Model file for the job. Use its own axes, mm. Face numbers are marked on the shaded views. A direction names the side the tool comes from. Give positions to 0.01 mm unless a question says otherwise; leave off trailing zeros. Loops run counter-clockwise (first coordinate to the right, second up) from the corner with the lowest first, then second, coordinate; pieces in that order, holes last. Notation, with made-up numbers: M 19.5,-31 L 46.5,-31 A9 ccw 46.5,-21 Z; hole C 3,-18 d6. An arc over 180 degrees is marked long. Answer in a Markdown table with one row per item.
Autodesk Inventor part; units mm, degrees
ref_plane "YZ Plane" through (0, 0, 0) normal (1, 0, 0) x (0, 1, 0)
ref_plane "XZ Plane" through (0, 0, 0) normal (0, 1, 0) x (-1, 0, 0)
ref_plane "XY Plane" through (0, 0, 0) normal (0, 0, 1) x (1, 0, 0)
sketch "Sketch1" plane through (0, 0, 0) normal (0, 1, 0) x (-1, 0, 0)
  line L0 (-10, 10) -> (10, 10)
  line L1 (10, 10) -> (10, -10)
  line L2 (10, -10) -> (-10, -10)
  line L3 (-10, -10) -> (-10, 10)
  line L4 (-10, 10) -> (10, -10) construction
  line L5 (10, 10) -> (-10, -10) construction
  point P0 (0, 0)
  dimension "d0" = 20
  dimension "d1" = 20
extrude "Extrusion1" add sketch "Sketch1" along normal blind 20
sketch "Sketch2" plane through (0, 20, 0) normal (0, 1, 0) x (1, 0, 0)
  line L0 (8.5, -8.5) -> (-8.5, -8.5)
  line L1 (-8.5, -8.5) -> (-8.5, 8.5)
  line L2 (-8.5, 8.5) -> (8.5, 8.5)
  line L3 (8.5, 8.5) -> (8.5, -8.5)
  line L4 (8.5, -8.5) -> (-8.5, 8.5) construction
  line L5 (-8.5, -8.5) -> (8.5, 8.5) construction
  point P0 (0, 0)
  dimension "d4" = 17
  dimension "d5" = 17
extrude "Extrusion2" cut sketch "Sketch2" against normal blind 17
sketch "Sketch6" plane through (-10, 0, 10) normal (0, 0, 1) x (1, 0, 0)
  line L0 (20, 0) -> (0, 0)
  line L1 (0, 20) -> (20, 0)
  line L2 (20, 0) -> (20, 20)
  line L3 (20, 20) -> (0, 20)
  line L4 (1.5, 20) -> (18.5, 20)
  point P0 (10, 0)
extrude "Extrusion6" cut sketch "Sketch6" against normal through all
sketch "Sketch7" plane through (0, 3, 0) normal (0, 1, 0) x (1, 0, 0)
  circle A0 centre (0, 0) radius 4.5
  dimension "d20" = 9
sketch "Sketch8" plane through (-8.5, 3, 8.5) normal (1, 0, 0) x (0, 0, -1)
  circle A0 centre (8.5, 8) radius 4.5
  line L0 (0, 0) -> (17, 0)
  point P0 (8.5, -3)
  dimension "d18" = 8
  dimension "d19" = 9
extrude "Extrusion7" cut sketch "Sketch8" against normal blind 10
extrude "Extrusion8" cut sketch "Sketch7" against normal blind 10
properties part number "corner bracket"
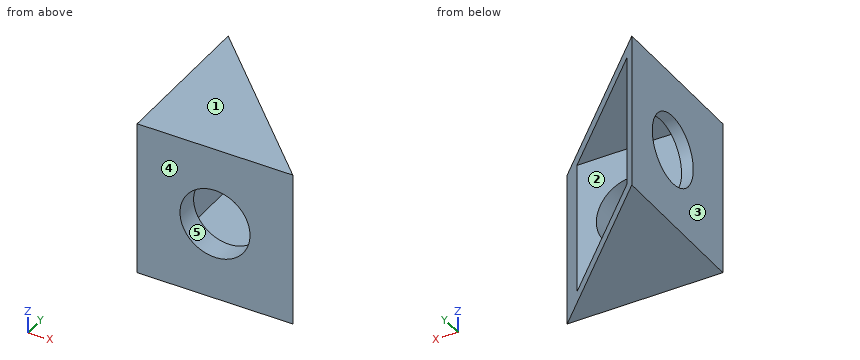
(1) Saw through at D-D, the plane x = 6.25. Give the cut face in (y, z).
Established:
| item | result |
|---|---|
| outline | M 0,-10 L 3.75,-10 L 3.75,-8.5 L 3,-8.5 L 3,8.5 L 3.75,8.5 L 3.75,10 L 0,10 Z |
(2) Saw through at C-C, the plane x = 0. Give the cut face in (y, z), and give its area (3 significant figures).
Established:
| item | result |
|---|---|
| outline | M 0,-10 L 10,-10 L 10,-8.5 L 3,-8.5 L 3,-4.5 L 0,-4.5 Z; M 0,4.5 L 3,4.5 L 3,8.5 L 10,8.5 L 10,10 L 0,10 Z |
| area | 54.0 mm2 |
(3) Flat gauge pins, fed straight in: P1, Ø1.5, axis at y = 7, z = 5, coming from the +X side; P2, Ø1.5, axis at x = 4.5, z = -6, coming from the +Y side. Where does each tip first touch, or does it go through?
Established:
| item | result |
|---|---|
| P1 | stops at x = -8.5 |
| P2 | stops at y = 3 |
(4) Wall check: L1, parallel to Z at x = 0, y = 1.45; L2, parallel to Z at x = 3.75, y = 4.75; L3, parallel to X at y = 4.75, z = 4. Give the ranges that are in metal, low to high.
Established:
| item | result |
|---|---|
| L1 | z = -10 to -4.5, 4.5 to 10 |
| L2 | z = -10 to -8.5, 8.5 to 10 |
| L3 | x = -10 to -8.5 |
(5) Saw through at B-B, the plane z = 0. Give the cut face in (x, y), and give its area (3 significant figures).
Established:
| item | result |
|---|---|
| outline | M -10,0 L -4.5,0 L -4.5,3 L -8.5,3 L -8.5,6.5 L -10,6.5 Z; M -10,15.5 L -8.5,15.5 L -8.5,18.5 L -10,20 Z; M 4.5,0 L 10,0 L 7,3 L 4.5,3 Z |
| area | 39.4 mm2 |
(6) Saw through at A-A, the plane y = 11. Give the cut face in (x, z).
Established:
| item | result |
|---|---|
| outline | M -10,-10 L -1,-10 L -1,-8.5 L -8.5,-8.5 L -8.5,-4.5 L -10,-4.5 Z; M -10,4.5 L -8.5,4.5 L -8.5,8.5 L -1,8.5 L -1,10 L -10,10 Z |
(7) Mould opens along X. For the marked faces 3, 4 and 5 say: pulls with the +X half, pulls with the -X half, needs draft (parallel to the pull), parting line crosses it, or undercut.
Established:
| item | result |
|---|---|
| face 3 | pulls with the -X half |
| face 4 | needs draft |
| face 5 | undercut |
(8) Which spindle directions (+Z, -Z, +X, -X, +Y, -Y) get a long thin tool onto all of the face, cutting with end or side? Do the marked faces 1 and 2. Say none if no direction does.
Established:
| item | result |
|---|---|
| face 1 | +Z, +X, -X, +Y, -Y |
| face 2 | +X, +Y |
